Autodesk Inventor part; units mm, degrees
ref_plane "YZ Plane" through (0, 0, 0) normal (1, 0, 0) x (0, 1, 0)
ref_plane "XZ Plane" through (0, 0, 0) normal (0, 1, 0) x (-1, 0, 0)
ref_plane "XY Plane" through (0, 0, 0) normal (0, 0, 1) x (1, 0, 0)
sketch "Sketch1" plane through (0, 0, 0) normal (0, 0, 1) x (1, 0, 0)
  line L0 (40.6435, -29.4735) -> (-71.3565, -29.4735)
  line L1 (-71.3565, -29.4735) -> (-71.3565, 48.5265)
  line L2 (40.6435, -29.4735) -> (40.6435, 2.5265)
  line L3 (40.6435, 2.5265) -> (17.6435, 48.5265)
  line L4 (17.6435, 48.5265) -> (-71.3565, 48.5265)
  point P0 (0, 0)
  point P1 (40.6435, 100.5706)
  dimension "d0" = 112
  dimension "d1" = 78
  dimension "d5" = 32
  dimension "d8" = 23
extrude "Extrusion1" add sketch "Sketch1" against normal blind 20
sketch "Sketch2" plane through (0, 0, 0) normal (0, 0, 1) x (1, 0, 0)
  point P0 (0, 0)
ref_plane "Work Plane1" through (-71.3565, -29.4735, 0) normal (0, -1, 0) x (1, 0, 0)
sketch "Sketch3" plane through (-71.3565, -29.4735, 0) normal (0, -1, 0) x (1, 0, 0)
  line L0 (0, 0) -> (0, 58)
  line L1 (0, 58) -> (42, 58)
  line L2 (42, 58) -> (42, 48)
  line L3 (42, 48) -> (104, 0)
  line L4 (112, 0) -> (89, 0)
  line L5 (0, 0) -> (104, 0)
  point P0 (71.3565, 0)
  dimension "d12" = 8
  dimension "d13" = 10
  dimension "d14" = 58
  dimension "d21" = 42
extrude "Extrusion2" add sketch "Sketch3" against normal blind 18
sketch "Sketch4" plane through (-71.3565, -29.4735, 0) normal (0, -1, 0) x (1, 0, 0)
  line L0 (0, 0) -> (0, 58)
  line L1 (0, 0) -> (32, 0)
  line L2 (32, 0) -> (32, 12)
  line L3 (32, 12) -> (0, 12)
  line L4 (0, 12) -> (0, 0)
  point P0 (71.3565, 0)
  point P1 (0, 12)
  dimension "d17" = 12
  dimension "d18" = 32
extrude "Extrusion3" add sketch "Sketch4" along normal blind 42
sketch "Sketch5" plane through (-71.3565, -11.4735, 0) normal (0, 1, 0) x (1, 0, 0)
  point P0 (71.3565, 0)
sketch "Sketch6" plane through (-71.3565, -11.4735, 0) normal (0, 1, 0) x (1, 0, 0)
  line L0 (42, -48) -> (104, 0)
  line L1 (0, -58) -> (42, -58)
  line L2 (0, -58) -> (42, -58)
  line L3 (42, -58) -> (42, -48)
  line L4 (42, -48) -> (104, 0)
  line L5 (0, 0) -> (104, 0)
  line L6 (0, 0) -> (0, -58)
  line L7 (0, 0) -> (0, -58)
  line L8 (42, -58) -> (42, -48)
  line L9 (0, -58) -> (0, -12)
  line L10 (42, -58) -> (0, -58)
  line L11 (0, -58) -> (0, -48)
  line L12 (0, -48) -> (42, -48)
  line L13 (42, -48) -> (42, -58)
  point P0 (71.3565, 0)
extrude "Extrusion4" add sketch "Sketch6" along normal blind 52 contours L3 L1 L6 L12
sketch "Sketch7" plane through (-71.3565, -29.4735, 12) normal (0, 0, 1) x (1, 0, 0)
  line L0 (0, 0) -> (0, -42)
  circle A0 centre (10, -31) radius 4
  circle A1 centre (20, -19) radius 4
  point P0 (71.3565, 29.4735)
  point P1 (10, -42)
  point P2 (0, -31)
  point P3 (20, -42)
  point P4 (0, -19)
  dimension "d24" = 10
  dimension "d25" = 11
  dimension "d26" = 8
  dimension "d27" = 20
  dimension "d28" = 23
  dimension "d29" = 8
extrude "Extrusion5" cut sketch "Sketch7" against normal blind 52
sketch "Sketch8" plane through (-71.3565, -29.4735, 58) normal (0, 0, 1) x (1, 0, 0)
  line L0 (42, 0) -> (0, 0)
  line L1 (42, 0) -> (42, 70)
  line L2 (0, 70) -> (42, 70)
  line L3 (0, 0) -> (0, 70)
  line L4 (0, 70) -> (42, 70)
  circle A0 centre (21, 50) radius 9
  point P0 (71.3565, 29.4735)
  point P1 (0, 50)
  point P2 (21, 70)
  point P3 (21, 70)
  dimension "d32" = 21
  dimension "d33" = 20
  dimension "d34" = 18
extrude "Extrusion6" cut sketch "Sketch8" against normal blind 20 contours A0
Verification items for the finished model (mm, model axes). A direction names the side the tool comes from. Give positions to 0.01 mm unless a question says otherwise; leave off trailing zeros. Order: outer loops, then holes, each group sorted by start corner. A loop starts at its lowest first (then second) coordinate and runs counter-clockwise, first axis right, second up. Notation, with made-up numbers: M 12.5,33.25 L 71.5,33.25 A29 ccw 71.5,58.25 Z; hole C -40,-34 d8. An arc over 180 degrees is marked long. Answer in a Markdown table with one row per item. Add a question column.
Item 1: Section check D-D, the plane y = 18. Enter the section's corners in (x, z), and give its area (3 significant figures).
Item 2: Gauge pin test, flat ends, axial feed: pin 1 (5 mm diameter, centred on y = -49, z = 4.5, fed in from +X); pin 2 (9 mm diameter, centred on x = -61.36, y = -60.47, fed in from +Z); pin 3 (5 mm diameter, centred on x = -58.5, z = 54.5, fed in from +Y). Record the tip position at first contact, or that the pin passes through.
Item 3: Section check C-C, the plane x = -43. Enter the section's corners in (y, z).
Item 4: Tool access check on faces 4 (the flat face through (-51, 40.526, 53)), 5 (the flat face through (-32, -11.474, 19)), 6 (the cylindrical face through (-46.204, 12.542, 53.07)). Record the directions out of +Z, -Z, +X, -X, +Y, -Y that give a thin tool (end or side, any length) a straight path to the whole face; none if there is none.
Item 5: Mould release check, pull along X, two halves, no side actions. Record for faces 1 (the flat face through (-39.356, -50, 6)), 2 (the flat face through (-27, -29.474, 11)), 3 (the cylindrical face through (-61.877, -56.508, 6.084)): released by +X, released by -X, zero draft, split by the parting line, or undercut.
Item 6: Section check B-B, the plane y = 1. Enter the section's corners in (x, z), and give its area (3 significant figures).
Item 7: Scan lines: probe 1 along Z at (x, y) = (-37.5, -4); probe 2 along Z at (x, y) = (17, 25.5); probe 3 along Y at (x, z) = (-44, 29.5). Record each from-to range of solid material in increasing order. Write a range as from..to.
Item 8: Section check A-A, the plane y = -16. Enter the section's corners in (x, z), and give its area (3 significant figures).
Filled sheet:
| question | item | result |
|---|---|---|
| 1 | outline | M -71.36,-20 L 32.91,-20 L 32.91,0 L -71.36,0 Z; M -71.36,48 L -58.99,48 L -58.99,58 L -71.36,58 Z; M -41.72,48 L -29.36,48 L -29.36,58 L -41.72,58 Z |
| 1 | area | 2,330 mm^2 |
| 2 | pin 1 | stops at x = -39.36 |
| 2 | pin 2 | stops at z = 12 |
| 2 | pin 3 | stops at y = 40.53 |
| 3 | outline | M -71.47,0 L -29.47,0 L -29.47,-20 L 48.53,-20 L 48.53,0 L -11.47,0 L -11.47,48 L 15.34,48 L 15.34,58 L -29.47,58 L -29.47,12 L -71.47,12 Z; M 25.71,48 L 40.53,48 L 40.53,58 L 25.71,58 Z |
| 4 | face 4 | +Z, +X, -X, +Y |
| 4 | face 5 | +X, -X, +Y |
| 4 | face 6 | +Z |
| 5 | face 1 | released by +X |
| 5 | face 2 | zero draft |
| 5 | face 3 | undercut |
| 6 | outline | M -71.36,-20 L 40.64,-20 L 40.64,0 L -71.36,0 Z; M -71.36,48 L -29.36,48 L -29.36,58 L -71.36,58 Z |
| 6 | area | 2,660 mm^2 |
| 7 | probe 1 | z = -20..0, 48..58 |
| 7 | probe 2 | z = -20..0 |
| 7 | probe 3 | y = -29.47..-11.47 |
| 8 | outline | M -71.36,-20 L 40.64,-20 L 40.64,0 L 32.64,0 L -29.36,48 L -29.36,58 L -71.36,58 Z |
| 8 | area | 6,160 mm^2 |
